from build123d import *

# Parameters (mm, degrees)
SKETCH1_W                  = 150
SKETCH1_H                  = 108
BOSS_EXTRUDE1_DEPTH        = 10
M6_TAPPED_HOLE1_AT_2_COUNT = 2
M6_TAPPED_HOLE1_AT_2_PITCH = 40
FILLET1_R                  = 10


with BuildPart() as part:
    # Sketch1 → Boss-Extrude1 (new body)
    with BuildSketch(Plane.XY):
        Rectangle(SKETCH1_W, SKETCH1_H)
    extrude(amount=BOSS_EXTRUDE1_DEPTH)

    # Sketch4 → M6 Tapped Hole1 (revolve, cut)
    with BuildSketch(Plane(origin=(-44.997893633, 20, 10), x_dir=(0, -1, 0), z_dir=(1, 0, 0))):
        Polygon((0, 0), (0, 16.502151548), (2.5, 15), (2.5, 0), align=None)
    m6_tapped_hole1 = revolve(axis=Axis((-44.997893633, 20, 16.35), (0, 0, -1)), mode=Mode.SUBTRACT)

    # M6 Tapped Hole1 at 2: M6 Tapped Hole1 ×2
    with Locations(*[(0, -i * M6_TAPPED_HOLE1_AT_2_PITCH, 0) for i in range(1, M6_TAPPED_HOLE1_AT_2_COUNT)]):
        add(m6_tapped_hole1, mode=Mode.SUBTRACT)

    # Mirror1: M6 Tapped Hole1 across plane
    add(m6_tapped_hole1.mirror(Plane(origin=(0, 0, 0), x_dir=(0, 0, 1), z_dir=(1, 0, 0))), mode=Mode.SUBTRACT)

    # Mirror1 copy 1 sketch → Mirror1 copy 1 (revolve, cut)
    with BuildSketch(Plane(origin=(44.997893633, -20, 10), x_dir=(0, -1, 0), z_dir=(-1, 0, 0))):
        Polygon((0, 0), (0, -16.502151548), (2.5, -15), (2.5, 0), align=None)
    revolve(axis=Axis((44.997893633, -20, 16.35), (0, 0, 1)), mode=Mode.SUBTRACT)

    # Fillet1
    fillet1_edges = [part.edges().sort_by_distance(p)[0] for p in [
        (75, -54, 5),
        (-75, -54, 5),
        (-75, 54, 5),
        (75, 54, 5),
    ]]
    fillet(fillet1_edges, radius=FILLET1_R)


solid = part.part
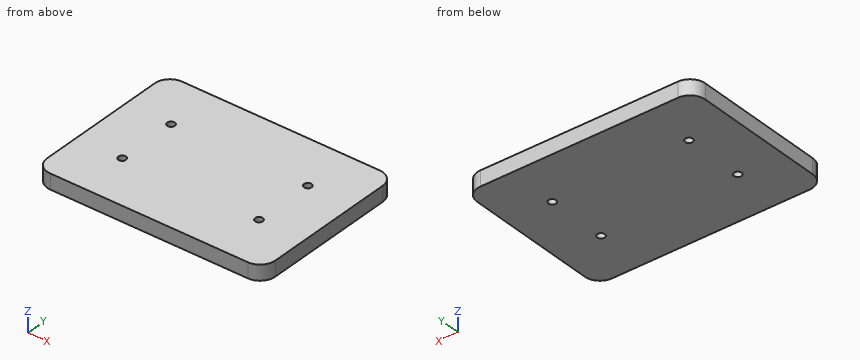
The model under review builds one solid part; all positions refer to its coordinate system, in mm. Coordinates: 2 decimals unless noted, no trailing zeros. Loops run counter-clockwise (first coordinate to the right, second up) from the corner with the lowest first, then second, coordinate; pieces in that order, holes last. Notation, with made-up numbers: (78, 3.5) -> (95, 3.5) arc R20 ccw to (95, 31.5) -> close; hole circle Ø5 at (-30.5, -38). An arc over 180 degrees is marked (long way). Use a Markdown table: item, result. Add a question column.
1. Add section A-A on y = -20. Write out the cut boundary in (x, z).
2. Clearance check with a flat-ended pin moving along its axis: pin 1 Ø3 at (x, y) = (45, -20) entering from +Z. State where the tip first meets the part, or that it passes through.
3. To check wall thickness, follow line 1 (X direction, y = -20, z = 3.5); line 2 (Y direction, x = -44, z = 1.5); line 3 (Y direction, x = -43, z = 9.5). State the ranges of each line that lie inside material, in increasing order.
Returned:
| question | item | result |
|---|---|---|
| 1 | outline | (-75, 0) -> (-47.5, 0) -> (-47.5, 10) -> (-75, 10) -> close; (-42.5, 0) -> (42.5, 0) -> (42.5, 10) -> (-42.5, 10) -> close; (47.5, 0) -> (75, 0) -> (75, 10) -> (47.5, 10) -> close |
| 2 | pin 1 | passes through |
| 3 | line 1 | x = -75 to -47.5, -42.5 to 42.5, 47.5 to 75 |
| 3 | line 2 | y = -54 to -22.29, -17.71 to 17.71, 22.29 to 54 |
| 3 | line 3 | y = -54 to -21.5, -18.5 to 18.5, 21.5 to 54 |
